Check sheet for the modelled part. Datum: model origin and axes. Units: mm. A direction names the side the tool comes from. Give positions to 0.01 mm unless a question says otherwise; leave off trailing zeros. Write each loop counter-clockwise with the first axis right and the second up, starting at its lowest first coordinate (ties: lowest second). Pieces come first, ordered by that corner, then holes. Notation, with made-up numbers: (7.5, -22.5) -> (59.5, -22.5) arc R12 cw to (59.5, -14.5) -> close; hole circle Ø8 at (43, 35.5). An arc over 180 degrees is marked (long way). Answer as a JSON object with one key per item and string values.
from build123d import *

# Parameters (mm, degrees)
SKETCH_1_R      = 12.5
EXTRUDE_1_DEPTH = 11


with BuildPart() as part:
    # 草图1 → 凸台-拉伸1 (new, symmetric)
    with BuildSketch(Plane.XY):
        with BuildLine():
            ThreePointArc((10, 2.638593384), (0, 34.5), (-10, 2.638593384))
            Line((-10, 2.638593384), (-10, -7.5))
            Line((-10, -7.5), (10, -7.5))
            Line((10, -7.5), (10, 2.638593384))
        make_face()
        with Locations((0, 17)):
            Circle(SKETCH_1_R, mode=Mode.SUBTRACT)
    extrude(amount=EXTRUDE_1_DEPTH, both=True)


solid = part.part
1. Sectioned sample at A-A, the plane y = 17. Enter the section's corners in (x, z), plus the area to 3 significant figures.
Determined:
{"outline": "(-17.5, -11) -> (-12.5, -11) -> (-12.5, 11) -> (-17.5, 11) -> close; (12.5, -11) -> (17.5, -11) -> (17.5, 11) -> (12.5, 11) -> close", "area": "220 mm^2"}
2. Sectioned sample at C-C, the plane z = 3. Enter the section's corners in (x, y).
Determined:
{"outline": "(-10, -7.5) -> (10, -7.5) -> (10, 2.64) arc R17.5 ccw (long way) to (-10, 2.64) -> close; hole circle Ø25 at (0, 17)"}
3. Go/stop test with flat-tipped pins: P1, Ø6, axis at y = 23.5, z = -7, coming from the +X side; P2, Ø10, axis at x = -14, z = 1, coming from the -Y side; P3, Ø8, axis at y = -2.5, z = -1, coming from the -X side; P4, Ø2, axis at x = -12, z = -5.5, coming from the +Y side. Record where each tip stops, or that it passes through.
Determined:
{"P1": "x = 17.15", "P2": "y = -7.5", "P3": "x = -10", "P4": "y = 30.61"}
4. Access from +Z, -Z, +X, -X, +Y, -Y to the whole of each face (thin tool, end or side, straight path). Record for faces 1 (the face through (0, 4, 11)), 2 (the face through (-10, -2, 0)).
Determined:
{"face 1": "+Z, +X, -X, +Y, -Y", "face 2": "+Z, -Z, -X, -Y"}
5. Sectioned sample at B-B, the plane x = 0. Enter the section's corners in (y, z), plus the area to 3 significant figures.
Determined:
{"outline": "(-7.5, -11) -> (4.5, -11) -> (4.5, 11) -> (-7.5, 11) -> close; (29.5, -11) -> (34.5, -11) -> (34.5, 11) -> (29.5, 11) -> close", "area": "374 mm^2"}
6. Scan lines: L1, parallel to Y at x = 0, z = -6; L2, parallel to X at y = 15, z = -10; L3, parallel to Y at x = 5, z = -8. Record each from-to range of solid material in increasing order. Write a range as [from, to].
Determined:
{"L1": "[-7.5, 4.5], [29.5, 34.5]", "L2": "[-17.39, -12.34], [12.34, 17.39]", "L3": "[-7.5, 5.54], [28.46, 33.77]"}
7. Sectioned sample at D-D, the plane y = -3. Enter the section's corners in (x, z), plus the area to 3 significant figures.
Determined:
{"outline": "(-10, -11) -> (10, -11) -> (10, 11) -> (-10, 11) -> close", "area": "440 mm^2"}
8. Mould release check, pull along Y, two halves, no side actions. Record for faces 3 (the face through (0.62, 34.49, 0.15)), 4 (the face through (5.77, 5.91, -0.15)), 5 (the face through (10, -3, 0)), 6 (the face through (0, -7.5, 0)): released by +Y, released by -Y, zero draft, split by the parting line, or undercut.
Determined:
{"face 3": "split by the parting line", "face 4": "undercut", "face 5": "zero draft", "face 6": "released by -Y"}
